Design review of the part built by this model. Coordinates are the model's own, in mm. A direction names the side the tool comes from. Coordinates: 2 decimals unless noted, no trailing zeros. Write each loop counter-clockwise with the first axis right and the second up, starting at its lowest first coordinate (ties: lowest second). Pieces come first, ordered by that corner, then holes.
Q1. Clearance check with flat-ended pins moving along their axes: pin 1 Ø6 at (x, y) = (18, 33.5) entering from -Z; pin 2 Ø4 at (x, z) = (14, 15) entering from +Y; pin 3 Ø1.8 at (x, z) = (23.75, 44) entering from -Y; pin 4 Ø8 at (x, y) = (12, 24.5) entering from +Z. State where each tip first meets the part, or that it passes through.
Q2. To check wall thickness, follow probe 1 along Z at (x, y) = (2.25, 2.5); probe 2 along Z at (x, y) = (14.5, 54.5); probe 3 along Y at (x, z) = (24.25, 32.5). State the ranges of each line that lie inside material, in increasing order.
Q3. Add section A-A, the plane y = 7.5. Give the boundary of the cut face in (x, z).
Q4. The part is to be moulded in two halves that separate along Z. For faces 1 (the face through (13, 2, 39)), 2 (the face through (10, 1, 48)), 3 (the face through (24.86, 6.08, 19.01)), 4 (the face through (2.31, 58.52, 5.67)), say which applies: +Z half, -Z half, draft (parallel to the pull), parting line (faces both ways), or undercut.
Q5. Add section B-B, the plane z = 44. Give the boundary of the cut face in (x, y).
Q6. Machinability: for faces 5 (the face through (24.2, 58.5, 6.1)), 6 (the face through (13.192, 7.07, 30.252)), 7 (the face through (13, 59, 10)), which of the approach directions +Z, -Z, +X, -X, +Y, -Y give a long, thin tool a straight path to every point of the face, cutting with its end or side? Answer none if there is none.
Q7. Add section D-D, the plane z = 7. Give the boundary of the cut face in (x, y).
Q8. Add section C-C, the plane x = 13. Give the boundary of the cut face in (y, z), plus the area to 4 significant figures.
Autodesk Fusion 360 part; units mm, degrees
sketch "Sketch1" plane through (0, 0, 0) normal (0, 0, 1) x (1, 0, 0)
  line L0 (0, 0) -> (26, 0)
  line L1 (26, 0) -> (26, 60)
  line L2 (26, 60) -> (0, 60)
  line L3 (0, 60) -> (0, 0)
  line L4 (0, 0) -> (26, 0)
  line L5 (26, 0) -> (26, 12)
  line L6 (26, 12) -> (0, 12)
  line L7 (0, 12) -> (0, 0)
  line L8 (0, 60) -> (26, 60)
  line L9 (26, 60) -> (26, 57)
  line L10 (26, 57) -> (0, 57)
  line L11 (0, 57) -> (0, 60)
  dimension "d1" = 26
  dimension "d2" = 60
  dimension "d16" = 48
  dimension "d43" = 3
extrude "Extrude1" add sketch "Sketch1" along normal blind 4 contours L1 L3 L6 L10
extrude "Extrude2" add sketch "Sketch1" along normal blind 48 contours L0 L1 L3 L4 L5 L6 L7
extrude "Extrude6" add sketch "Sketch1" along normal blind 10 contours L1 L2 L3 L8 L9 L10 L11
sketch "Sketch2" plane through (0, 12, 0) normal (0, 1, 0) x (-1, 0, 0)
  line L0 (-26, 4) -> (0, 4)
  line L1 (0, 4) -> (0, 48)
  line L2 (0, 48) -> (-26, 48)
  line L3 (-26, 48) -> (-26, 4)
  circle A0 centre (-13, 39) radius 8.75
  line L4 (-21.75, 39) -> (-21.75, 48)
  line L5 (-4.25, 39) -> (-4.25, 48)
  dimension "d17" = 17.5
  dimension "d27" = 13
  dimension "d28" = 4.25
  dimension "d46" = 35
extrude "Extrude3" cut sketch "Sketch2" against normal blind 10 contours L2 A0 L4 L5 | A0
sketch "Sketch3" plane through (0, 12, 0) normal (0, 1, 0) x (-1, 0, 0)
  line L0 (-26, 4) -> (0, 4)
  line L1 (0, 4) -> (0, 48)
  line L2 (-21.75, 48) -> (-26, 48)
  line L3 (-26, 48) -> (-26, 4)
  line L4 (-21.75, 39) -> (-21.75, 48)
  line L5 (0, 48) -> (-4.25, 48)
  line L6 (-4.25, 48) -> (-4.25, 39)
  arc A0 (-21.75, 39) -> (-4.25, 39) centre (-13, 39) ccw
  circle A1 centre (-23.75, 44) radius 1.5
  circle A2 centre (-2.25, 44) radius 1.5
  circle A3 centre (-23.75, 18) radius 1.5
  circle A4 centre (-2.25, 18) radius 1.5
  dimension "d29" = 3
  dimension "d30" = 2.25
  dimension "d31" = 3
  dimension "d32" = 2.25
  dimension "d33" = 3
  dimension "d34" = 3
  dimension "d35" = 2.25
  dimension "d36" = 2.25
  dimension "d37" = 4
  dimension "d38" = 4
  dimension "d57" = 30
  dimension "d58" = 30
extrude "Extrude5" cut sketch "Sketch3" against normal blind 13 contours A1 | A2 | A3 | A4
sketch "Sketch4" plane through (0, 60, 0) normal (0, 1, 0) x (-1, 0, 0)
  line L0 (-26, 0) -> (0, 0)
  line L1 (0, 0) -> (0, 10)
  line L2 (0, 10) -> (-26, 10)
  line L3 (-26, 10) -> (-26, 0)
  circle A0 centre (-3, 7) radius 1.5
  circle A1 centre (-23, 7) radius 1.5
  dimension "d49" = 3
  dimension "d50" = 3
  dimension "d51" = 3
  dimension "d52" = 3
  dimension "d53" = 3
  dimension "d54" = 3
extrude "Extrude7" cut sketch "Sketch4" against normal blind 4 contours A0 | A1
Here are the results:
1. pin 1: stops at z = 0
1. pin 2: stops at y = 12
1. pin 3: passes through
1. pin 4: stops at z = 4
2. probe 1: z = 0 to 16.5, 19.5 to 42.5, 45.5 to 48
2. probe 2: z = 0 to 4
2. probe 3: y = 0 to 12
3. outline: (0, 0) - (26, 0) - (26, 48) - (21.75, 48) - (21.75, 39) arc R8.75 cw to (4.25, 39) - (4.25, 48) - (0, 48) - close; hole circle Ø3 at (2.25, 18); hole circle Ø3 at (2.25, 44); hole circle Ø3 at (23.75, 18); hole circle Ø3 at (23.75, 44)
4. face 1: draft
4. face 2: +Z half
4. face 3: undercut
4. face 4: undercut
5. outline: (0, 0) - (0.75, 0) - (0.75, 12) - (0, 12) - close; (3.75, 0) - (22.25, 0) - (22.25, 12) - (21.75, 12) - (21.75, 2) - (4.25, 2) - (4.25, 12) - (3.75, 12) - close; (25.25, 0) - (26, 0) - (26, 12) - (25.25, 12) - close
6. face 5: +Y
6. face 6: +Z, +Y
6. face 7: +Z, +X, -X, +Y
7. outline: (0, 0) - (26, 0) - (26, 12) - (0, 12) - close; (0, 57) - (1.5, 57) - (1.5, 60) - (0, 60) - close; (4.5, 57) - (21.5, 57) - (21.5, 60) - (4.5, 60) - close; (24.5, 57) - (26, 57) - (26, 60) - (24.5, 60) - close
8. outline: (0, 0) - (60, 0) - (60, 10) - (57, 10) - (57, 4) - (12, 4) - (12, 30.25) - (2, 30.25) - (2, 48) - (0, 48) - close
8. area: 608.5 mm2
